CAD build for the part. Positions are in the model's coordinates, mm. Face numbers are marked on the shaded views. Give positions to 0.01 mm unless a question says otherwise; leave off trailing zeros. Order: outer loops, then holes, each group sorted by start corner. A loop starts at its lowest first (then second) coordinate and runs counter-clockwise, first axis right, second up. Notation, with made-up numbers: (88, -9.75) -> (111, -9.75) arc R8 ccw to (111, -0.75) -> close; hole circle Ø2 at (27, 42.25). An arc over 180 degrees is marked (long way). Answer as CSV lines item,"result".
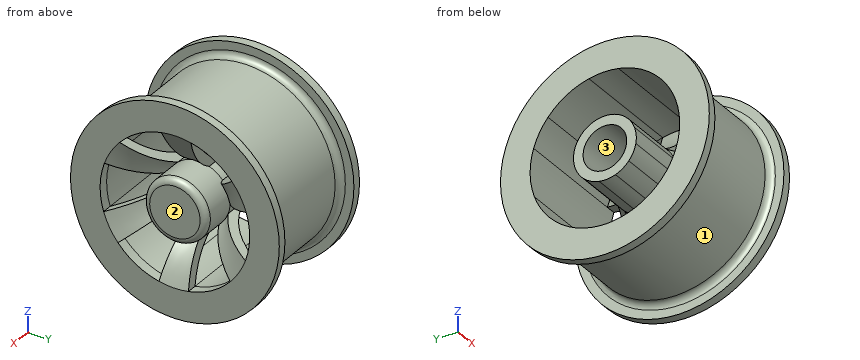
```python
from build123d import *
from build123d.topology import SkipClean

# Parameters (mm, degrees)
SKETCH2_R           = 12.812507943
SKETCH2_R_2         = 8.89
BOSS_EXTRUDE1_DEPTH = 50.8
SKETCH3_R           = 12.812507943
BOSS_EXTRUDE2_DEPTH = 10.16
CUT_EXTRUDE1_DEPTH  = 79.745120801
CIRPATTERN1_COUNT   = 6
FILLET1_R           = 2.54


# Read off the part's stored shape, not the designer's step: Revolve1
with BuildPart() as part:
    # Revolve1 outline → Revolve1 (revolve)
    with BuildSketch(Plane.YX):
        with BuildLine():
            Line((8.89, 0), (12.812507943, 0))
            add(Edge.make_bspline(
                [(30.48, 21.267937651), (30.309023597, 21.192105008), (29.508904573, 20.830209988), (27.54071299, 19.853128917), (24.775190006, 18.16464464), (21.854472712, 15.840046365), (19.302035246, 13.206553615), (17.10058625, 10.247215331), (15.23937391, 6.941426723), (13.969670275, 3.872573278), (13.216678126, 1.508927527), (12.91724489, 0.408653288), (12.812507943, 0)],
                knots=[0.045662691, 0.045662691, 0.045662691, 0.045662691, 0.0625, 0.125, 0.25, 0.375, 0.5, 0.625, 0.75, 0.875, 0.9375, 0.974110002, 0.974110002, 0.974110002, 0.974110002], degree=3))
            Line((30.48, 21.267937651), (30.48, -25.4))
            Line((30.48, -25.4), (42.545, -25.4))
            Line((42.545, -25.4), (42.545, -21.844))
            Line((42.545, -21.844), (39.0525, -21.844))
            ThreePointArc((39.0525, -21.844), (37.256448776, -21.100051224), (36.5125, -19.304))
            Line((36.5125, -19.304), (36.5125, 19.304))
            ThreePointArc((36.5125, 19.304), (37.256448776, 21.100051224), (39.0525, 21.844))
            Line((39.0525, 21.844), (42.545, 21.844))
            Line((42.545, 21.844), (42.545, 25.4))
            Line((42.545, 25.4), (30.48, 25.4))
            add(Edge.make_bspline(
                [(30.48, 25.4), (13.230283967, 18.539405633), (8.89, 0)],
                knots=[0.751440896, 0.751440896, 0.751440896, 1.751440896, 1.751440896, 1.751440896], degree=2))
        make_face()
    revolve(axis=Axis((0, 0, 0), (1, 0, 0)))



with BuildPart() as body_2:
    # Sketch2 → Boss-Extrude1 (new body)
    with BuildSketch(Plane.ZY.offset(25.4)):
        Circle(SKETCH2_R)
        Circle(SKETCH2_R_2, mode=Mode.SUBTRACT)
    extrude(amount=-BOSS_EXTRUDE1_DEPTH)


with BuildPart() as part_1:
    add(part.part)

    add(body_2.part)  # Boss-Extrude2 merges body 2
    # Sketch3 → Boss-Extrude2 (add)
    with BuildSketch(Plane(origin=(25.4, 0, 0), x_dir=(0, 0, -1), z_dir=(1, 0, 0))):
        with Locations(Location((0, 0, 0), (0, 0, 180))):
            Circle(SKETCH3_R)
    extrude(amount=-BOSS_EXTRUDE2_DEPTH)

    # Sketch4 → Cut-Extrude1 (cut, through all)
    with BuildSketch(Plane(origin=(25.4, 0, 0), x_dir=(0, 0, -1), z_dir=(1, 0, 0))):
        with BuildLine():
            Line((-9.243384813, 29.044624928), (-2.296598789, 12.604998762))
            ThreePointArc((-2.296598789, 12.604998762), (1.031106032, 12.770950636), (4.289083469, 12.07328136))
            Line((4.289083469, 12.07328136), (10.203409411, 28.721435138))
            ThreePointArc((10.203409411, 28.721435138), (0.506482692, 30.475791627), (-9.243384813, 29.044624928))
        make_face()
    cut_extrude1 = extrude(amount=-CUT_EXTRUDE1_DEPTH, mode=Mode.SUBTRACT)

    # CirPattern1: Cut-Extrude1 ×6 about axis
    with SkipClean():  # the faces are left unmerged after this step: merging them gives an invalid solid
        cirpattern1_axis = Axis((0, 0, 0), (1, 0, 0))
        for i in range(1, CIRPATTERN1_COUNT):
            add(cut_extrude1.rotate(cirpattern1_axis, i * 360 / CIRPATTERN1_COUNT), mode=Mode.SUBTRACT)

    # Fillet1
    fillet1_edges = [part_1.edges().sort_by_distance(p)[0] for p in [
        (25.4, 12.027308376, 4.416357439),
    ]]
    fillet(fillet1_edges, radius=FILLET1_R)


solid = part_1.part
```
1) Band-saw the part on A-A, the plane z = 0. Give the number of separate pieces and of enclosed holes in the cut face, then the cut area to 3 significant figures.
Data:
separate pieces,"3"
enclosed holes,"0"
area,"1,280 mm2"
2) Pull direction Y, two halves, no side cores. Call the marked faces 1, 2 and 3: pulls with the +Y half, pulls with the -Y half, needs draft (parallel to the pull), parting line crosses it, or undercut.
Data:
face 1,"parting line crosses it"
face 2,"needs draft"
face 3,"undercut"
3) Pin check, flat tips, straight feed: P1, Ø8, axis at x = -8, y = 5.5, coming from the +Z side; P2, Ø3, axis at x = -3.5, y = 10, coming from the -Z side; P3, Ø12, axis at x = 13.5, z = -3.5, coming from the +Y side; P4, Ø4, axis at y = -10.5, z = -10, coming from the -X side. Stop position of each tip, or through.
Data:
P1,"stops at z = 36.48"
P2,"stops at z = -35.51"
P3,"stops at y = 36.51"
P4,"stops at x = -25.4"
4) Wall check: line 1 along Y through (x, z) = (-16, -0.5); line 2 along X through (y, z) = (29.5, 28.5); line 3 along Z through (x, y) = (14, -1.5). Give the ranges that are in metal, low to high. Write a range as [from, to].
Data:
line 1,"y = [-36.51, -30.48], [-12.8, -8.88], [8.88, 12.8], [30.48, 36.51]"
line 2,"x = [-25.4, -21.84], [21.84, 25.4]"
line 3,"z = [-36.48, -30.44], [-20.06, -15.09], [-12.72, -8.76], [8.76, 12.72], [15.09, 20.06], [30.44, 36.48]"
5) Band-saw the part on B-B, the plane x = -9. Write the cut outline in (y, z) (1 decimal), then the cut area to 3 significant figures.
Data:
outline,"circle Ø73 at (0, 0); circle Ø25.6 at (0, 0); hole circle Ø61 at (0, 0); hole circle Ø17.8 at (0, 0)"
area,"1,540 mm2"
